Part print with two shaded views. Sizes in mm from the minimum x, y, z corner. Coordinates: 2 decimals unless noted, no trailing zeros. Write each loop counter-clockwise with the first axis right and the second up, starting at its lowest first coordinate (ties: lowest second). Pieces come first, ordered by that corner, then holes. Notation, with made-up numbers: (22, 26.5) - (77, 26.5) arc R6 cw to (77, 31.5) - close; hole circle Ø9 at (6.25, 6). An arc over 180 degrees is marked (long way). Answer in a Markdown table with one row per item. Add a question column.
Q1. Drill centre lines: line 1 along X through (y, z) = (4.75, 10); line 2 along Y through (x, z) = (224.5, 8); line 3 along X through (y, z) = (11.25, 10). Where is each one in solid material? Low to high. Write a range as from..to.
Q2. Pin check, flat tips, straight feed: pin 1 (1.5 mm diameter, centred on x = 144.5, z = 17, fed in from -Y); pin 2 (5 mm diameter, centred on x = 40, z = 10, fed in from -Y). Stop position of each tip, or through.
Q3. Band-saw the part on C-C (z = 10). List the corners of the cut face in (x, y), and give its area (3 significant figures).
Q4. Band-saw the part on B-B (x = 224.5). List the corners of the cut face in (y, z), and give its area (3 significant figures).
Q5. Band-saw the part on A-A (y = 10). List the corners of the cut face in (x, z).
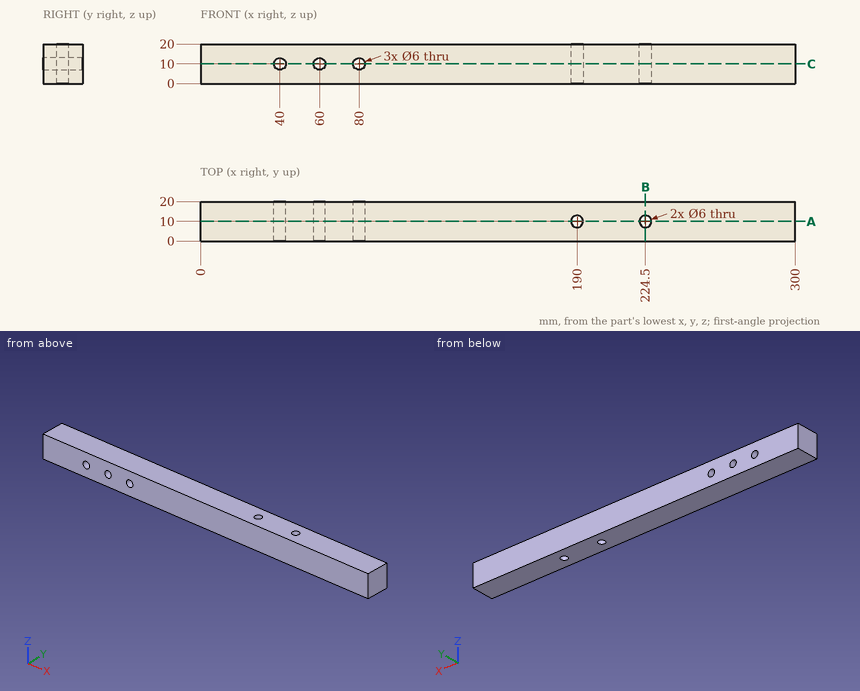
Checked values:
| question | item | result |
|---|---|---|
| 1 | line 1 | x = 0..37, 43..57, 63..77, 83..300 |
| 1 | line 2 | y = 0..7, 13..20 |
| 1 | line 3 | x = 0..37, 43..57, 63..77, 83..187.27, 192.73..221.77, 227.23..300 |
| 2 | pin 1 | stops at y = 0 |
| 2 | pin 2 | passes through |
| 3 | outline | (0, 0) - (37, 0) - (37, 20) - (0, 20) - close; (43, 0) - (57, 0) - (57, 20) - (43, 20) - close; (63, 0) - (77, 0) - (77, 20) - (63, 20) - close; (83, 0) - (300, 0) - (300, 20) - (83, 20) - close; hole circle Ø6 at (190, 10); hole circle Ø6 at (224.5, 10) |
| 3 | area | 5,580 mm² |
| 4 | outline | (0, 0) - (7, 0) - (7, 20) - (0, 20) - close; (13, 0) - (20, 0) - (20, 20) - (13, 20) - close |
| 4 | area | 280 mm² |
| 5 | outline | (0, 0) - (187, 0) - (187, 20) - (0, 20) - close; (193, 0) - (221.5, 0) - (221.5, 20) - (193, 20) - close; (227.5, 0) - (300, 0) - (300, 20) - (227.5, 20) - close; hole circle Ø6 at (40, 10); hole circle Ø6 at (60, 10); hole circle Ø6 at (80, 10) |
